```python
from build123d import *

# Parameters (mm, degrees)
SKETCH1_R             = 5.25
SKETCH1_R_2           = 3.25
BOSS_EXTRUDE1_DEPTH   = 9.2
BOSS_EXTRUDE1_2_DEPTH = 9.2
BOSS_EXTRUDE2_DEPTH   = 2
SKETCH3_W             = 2.5
SKETCH3_H             = 7.3
BOSS_EXTRUDE3_DEPTH   = 7.2
BOSS_EXTRUDE4_DEPTH   = 2
SKETCH6_R             = 0.25
BOSS_EXTRUDE5_DEPTH   = 7.2
BOSS_EXTRUDE6_REACH   = 27.811
SKETCH7_W             = 7.05
SKETCH7_H             = 1
FILLET3_R             = 3.45
FILLET4_DEPTH         = 2
FILLET4_2_DEPTH       = 2
FILLET4_START         = 2
FILLET4_3_DEPTH       = 0.883001
FILLET4_START_2       = 7.928754
FILLET4_4_DEPTH       = 3.171246
FILLET4_START_3       = 2.883001
FILLET4_5_DEPTH       = 2.866999


with BuildPart() as part:
    # Sketch1 → Boss-Extrude1 (new body)
    with BuildSketch(Plane(origin=(0, 0, 0), x_dir=(1, 0, 0), z_dir=(0, 1, 0))):
        with Locations(Location((-17, 0, 0), (0, 0, 270))):
            Circle(SKETCH1_R)
        with Locations(Location((-17, 0, 0), (0, 0, 270))):
            Circle(SKETCH1_R_2, mode=Mode.SUBTRACT)
    extrude(amount=BOSS_EXTRUDE1_DEPTH)



with BuildPart() as body_2:
    # Sketch1 → Boss-Extrude1 2 (new body)
    with BuildSketch(Plane(origin=(0, 0, 0), x_dir=(1, 0, 0), z_dir=(0, 1, 0))):
        with Locations(Location((17, 0, 0), (0, 0, 90))):
            Circle(SKETCH1_R)
        with Locations(Location((17, 0, 0), (0, 0, 90))):
            Circle(SKETCH1_R_2, mode=Mode.SUBTRACT)
    extrude(amount=BOSS_EXTRUDE1_2_DEPTH)


with BuildPart() as part_1:
    add(part.part)

    add(body_2.part)  # Boss-Extrude2 merges body 2
    # Sketch2 → Boss-Extrude2 (add)
    with BuildSketch(Plane(origin=(0, 0, 0), x_dir=(1, 0, 0), z_dir=(0, 1, 0))):
        with BuildLine():
            Line((17, 9.3), (-17, 9.3))
            Line((-17, 9.3), (-17, 3.25))
            ThreePointArc((-17, 3.25), (-15.574781, 2.92083), (-14.438262, 2))
            Line((-14.438262, 2), (14.438262, 2))
            ThreePointArc((14.438262, 2), (15.574781, 2.92083), (17, 3.25))
            Line((17, 3.25), (17, 9.3))
        make_face()
    extrude(amount=BOSS_EXTRUDE2_DEPTH)

    # Sketch3 → Boss-Extrude3 (add)
    with BuildSketch(Plane(origin=(0, 2, 0), x_dir=(1, 0, 0), z_dir=(0, 1, 0))):
        with Locations((0.3, 5.65)):
            Rectangle(SKETCH3_W, SKETCH3_H)
        with Locations((9.85, 5.65)):
            Rectangle(SKETCH3_W, SKETCH3_H)
    extrude(amount=BOSS_EXTRUDE3_DEPTH)

    # Sketch5 → Boss-Extrude4 (add)
    with BuildSketch(Plane(origin=(0, 9.2, 0), x_dir=(1, 0, 0), z_dir=(0, 1, 0))):
        with BuildLine():
            Line((1.55, 9.3), (-0.95, 9.3))
            Line((-0.95, 9.3), (-0.95, -1.45))
            Line((-0.95, -1.45), (9.1, -1.45))
            ThreePointArc((9.1, -1.45), (10.514214, -0.864214), (11.1, 0.55))
            Line((11.1, 0.55), (11.1, 2))
            Line((11.1, 2), (8.6, 2))
            Line((8.6, 2), (1.55, 2))
            Line((1.55, 2), (1.55, 9.3))
        make_face()
        with BuildLine():
            Line((8.6, 9.3), (8.6, 2))
            Line((8.6, 2), (11.1, 2))
            Line((11.1, 2), (11.1, 7.3))
            ThreePointArc((11.1, 7.3), (10.514214, 8.714214), (9.1, 9.3))
            Line((9.1, 9.3), (8.6, 9.3))
        make_face()
        with BuildLine():
            Line((2.325, 9.3), (1.55, 9.3))
            Line((1.55, 9.3), (1.55, 2))
            Line((1.55, 2), (8.6, 2))
            Line((8.6, 2), (8.6, 9.3))
            Line((8.6, 9.3), (7.825, 9.3))
            Line((7.825, 9.3), (7.825, 6.55))
            ThreePointArc((7.825, 6.55), (5.075, 3.8), (2.325, 6.55))
            Line((2.325, 6.55), (2.325, 9.3))
        make_face()
    extrude(amount=BOSS_EXTRUDE4_DEPTH)

    # Sketch6 → Boss-Extrude5 (add)
    with BuildSketch(Plane(origin=(0, 2, 0), x_dir=(1, 0, 0), z_dir=(0, 1, 0))):
        with Locations((1.55, 7.3)):
            Circle(SKETCH6_R)
        with Locations((1.55, 4)):
            Circle(SKETCH6_R)
        with Locations((8.6, 7.3)):
            Circle(SKETCH6_R)
        with Locations((8.6, 4)):
            Circle(SKETCH6_R)
    extrude(amount=BOSS_EXTRUDE5_DEPTH)

    # Sketch7 → Boss-Extrude6 (add, up to next)
    with BuildSketch(Plane(origin=(0, 2, 0), x_dir=(1, 0, 0), z_dir=(0, 1, 0)), mode=Mode.PRIVATE) as boss_extrude6_sk1:
        with Locations((5.075, 2.5)):
            Rectangle(SKETCH7_W, SKETCH7_H)
    boss_extrude6_tool1 = extrude(boss_extrude6_sk1.sketch, amount=BOSS_EXTRUDE6_REACH, mode=Mode.PRIVATE) - part_1.part
    add(boss_extrude6_tool1.solids().sort_by_distance((5.075, 2, -2.5))[0])

    # Fillet3
    fillet3_edges = [part_1.edges().sort_by_distance(p)[0] for p in [
        (5.075, 9.2, -2),
    ]]
    fillet(fillet3_edges, radius=FILLET3_R - 0.0001)  # a hair under: the kernel refuses the full size

    # Fillet4: read off the stored shape, not the designer's step
    # Fillet4 outline → Fillet4 (cut)
    with BuildSketch(Plane(origin=(0, 0, 0), x_dir=(1, 0, 0), z_dir=(0, 1, 0))):
        with BuildLine():
            ThreePointArc((12.95, 9.3), (15.813782, 8.113782), (17, 5.25))
            Line((17, 5.25), (17, 9.3))
            Line((17, 9.3), (12.95, 9.3))
        make_face()
        with BuildLine():
            ThreePointArc((-17, 5.25), (-15.813782, 8.113782), (-12.95, 9.3))
            Line((-12.95, 9.3), (-17, 9.3))
            Line((-17, 9.3), (-17, 5.25))
        make_face()
    extrude(amount=FILLET4_DEPTH, mode=Mode.SUBTRACT)

    # Fillet4 2 outline → Fillet4 2 (add)
    with BuildSketch(Plane(origin=(0, 0, 0), x_dir=(1, 0, 0), z_dir=(0, 1, 0))):
        with BuildLine():
            ThreePointArc((7.928754, 2), (10.457281, 1.113709), (11.879135, -1.157258))
            ThreePointArc((11.879135, -1.157258), (11.768637, 0.441974), (12.145878, 2))
            Line((12.145878, 2), (7.928754, 2))
        make_face()
        with BuildLine():
            ThreePointArc((-11.879135, -1.157258), (-10.457281, 1.113709), (-7.928754, 2))
            Line((-7.928754, 2), (-12.145878, 2))
            ThreePointArc((-12.145878, 2), (-11.768637, 0.441974), (-11.879135, -1.157258))
        make_face()
    extrude(amount=FILLET4_2_DEPTH)

    # Fillet4 3 outline → Fillet4 3 (add)
    with BuildSketch(Plane(origin=(0, 0, 0), x_dir=(1, 0, 0), z_dir=(0, 1, 0)).offset(FILLET4_START)):
        with BuildLine():
            ThreePointArc((7.928754, 2), (9.689475, 1.59724), (11.1, 0.469067))
            Line((11.1, 0.469067), (11.1, 2))
            Line((11.1, 2), (7.928754, 2))
        make_face()
    extrude(amount=FILLET4_3_DEPTH)

    # Fillet4 4 outline → Fillet4 4 (add)
    with BuildSketch(Plane.YZ.offset(FILLET4_START_2)):
        with BuildLine():
            ThreePointArc((5.75, -2), (4.124928, -1.593294), (2.883001, -0.469067))
            Line((2.883001, -0.469067), (2.883001, -2))
            Line((2.883001, -2), (5.75, -2))
        make_face()
    extrude(amount=FILLET4_4_DEPTH)

    # Fillet4 5 outline → Fillet4 5 (cut)
    with BuildSketch(Plane(origin=(0, 0, 0), x_dir=(1, 0, 0), z_dir=(0, 1, 0)).offset(FILLET4_START_3)):
        with BuildLine():
            ThreePointArc((11.840276, -1), (10.393506, 1.163643), (7.928754, 2))
            Line((7.928754, 2), (7.928754, -1))
            Line((7.928754, -1), (11.840276, -1))
        make_face()
    extrude(amount=FILLET4_5_DEPTH, mode=Mode.SUBTRACT)


solid = part_1.part
```
Source: CAD feature listing. Evaluate the final solid. Frame: model axes, mm. A direction names the side the tool comes from. Coordinates: 2 decimals unless noted, no trailing zeros. Loops run counter-clockwise (first coordinate to the right, second up) from the corner with the lowest first, then second, coordinate; pieces in that order, holes last. Notation, with made-up numbers: M 49.5,3.5 L 90.5,3.5 A18 cw 90.5,15.5 Z; hole C -32.5,76 d11. An arc over 180 degrees is marked long. Use a Markdown table: item, result. Add a question column.
Q1. Access query for faces 1 (the cylindrical face through (20.19, 4.54, 4.17)), 2 (the flat face through (1.55, 6, -6)), 3 (the flat face through (16.9, 9.2, -3.4)), 4 (the cylindrical face through (-10.487, 0.986, -1.09)), 5 (the cylindrical face through (10.53, 10.19, -8.7)). Directions: +Z, -Z, +X, -X, +Y, -Y. A direction counts if a zero-diameter tool reaches every point of the face in a straight line with its end or side. Return the directions, or none.
Q2. First-contact query: pin 1 (5 mm diameter, centred on x = 18, z = -2, fed in from +Y); pin 2 (2 mm diameter, centred on x = -6, y = 4.5, fed in from -Z); pin 3 (1.5 mm diameter, centred on x = 13.5, y = 7.5, fed in from +Z); pin 4 (5 mm diameter, centred on y = 7.5, z = -6.5, fed in from -X). Flat tips, straight axial feed; report the tip coordinate or a pass-through.
Q3. Draft query along Y for faces 6 (the flat face through (2.325, 10, -8)), 7 (the flat face through (10.6, 9.2, -8.9)), 8 (the flat face through (5, 6, -3)). Return one class per face: pulls with the +Y half, pulls with the -Y half, needs draft (parallel to the pull), parting line crosses it, or undercut.
Q4. Material intervals for L1, parallel to X at y = 5, z = 0; L2, parallel to Y at x = 2, z = -6.25; L3, parallel to Z at x = 17, y = 5.5, sorted ascending.
Q5. Section query D-D, the plane y = 8. Return loops of the section in (x, z), and give its area (3 significant figures).
Q6. Section query A-A, the plane y = 3.75. Return loops of the section in (x, z), and give its area (3 significant figures).
Q7. Section query C-C, the plane y = 1.25. Return loops of the section in (x, z).
Q8. Section query B-B, the plane z = 2. Return loops of the section in (x, y).
Result:
| question | item | result |
|---|---|---|
| 1 | face 1 | +Y |
| 1 | face 2 | none |
| 1 | face 3 | +Z, -Z, +X, +Y |
| 1 | face 4 | +Z, +Y, -Y |
| 1 | face 5 | -Z, +X, +Y |
| 2 | pin 1 | stops at y = 9.2 |
| 2 | pin 2 | passes through |
| 2 | pin 3 | stops at z = 4.47 |
| 2 | pin 4 | stops at x = -20.4 |
| 3 | face 6 | needs draft |
| 3 | face 7 | pulls with the +Y half |
| 3 | face 8 | undercut |
| 4 | L1 | x = -22.25 to -20.25, -13.75 to -11.75, 11.75 to 13.75, 20.25 to 22.25 |
| 4 | L2 | y = 0 to 2, 9.2 to 11.2 |
| 4 | L3 | z = -5.25 to -3.25, 3.25 to 5.25 |
| 5 | outline | C -17,0 d10.5; M -0.95,-9.3 L 1.55,-9.3 L 1.55,-7.55 A0.25 ccw 1.55,-7.05 L 1.55,-4.25 A0.25 ccw 1.55,-3.75 L 1.55,-3 L 8.6,-3 L 8.6,-3.75 A0.25 ccw 8.6,-4.25 L 8.6,-7.05 A0.25 ccw 8.6,-7.55 L 8.6,-9.3 L 11.1,-9.3 L 11.1,-1.17 L -0.95,-1.17 Z; C 17,0 d10.5; hole C -17,0 d6.5; hole C 17,0 d6.5 |
| 5 | area | 161 mm2 |
| 6 | outline | C -17,0 d10.5; M -0.95,-9.3 L 1.55,-9.3 L 1.55,-7.55 A0.25 ccw 1.55,-7.05 L 1.55,-4.25 A0.25 ccw 1.55,-3.75 L 1.55,-3 L 8.6,-3 L 8.6,-3.75 A0.25 ccw 8.6,-4.25 L 8.6,-7.05 A0.25 ccw 8.6,-7.55 L 8.6,-9.3 L 11.1,-9.3 L 11.1,-1.36 L 10.11,-1.36 A4.05 cw 7.93,-2 L -0.95,-2 Z; C 17,0 d10.5; hole C -17,0 d6.5; hole C 17,0 d6.5 |
| 6 | area | 152 mm2 |
| 7 | outline | M -17,-5.25 A4.05 ccw -12.95,-9.3 L 12.95,-9.3 A4.05 ccw 17,-5.25 A5.25 ccw long 11.88,1.16 A4.05 cw 7.93,-2 L -7.93,-2 A4.05 cw -11.88,1.16 A5.25 ccw long Z; hole M -17,-3.25 A3.25 ccw -14.44,-2 A3.25 ccw long Z; hole C 17,0 d6.5 |
| 8 | outline | M -21.85,0 L -19.56,0 L -19.56,9.2 L -21.85,9.2 Z; M -14.44,0 L -12.15,0 L -12.15,9.2 L -14.44,9.2 Z; M 12.15,0 L 14.44,0 L 14.44,9.2 L 12.15,9.2 Z; M 19.56,0 L 21.85,0 L 21.85,9.2 L 19.56,9.2 Z |
